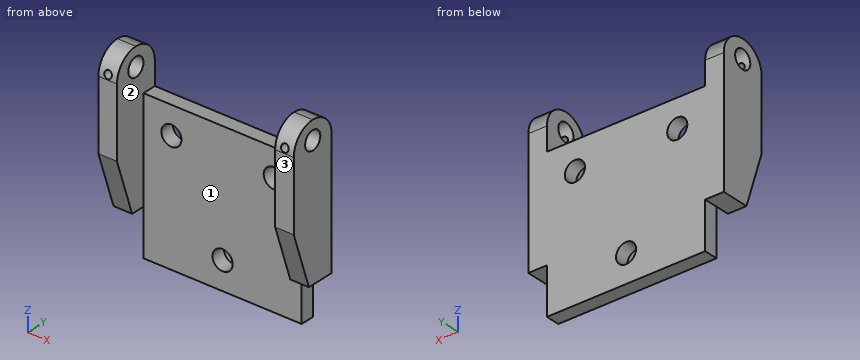
from build123d import *

# Parameters (mm, degrees)
F0_W         = 53.975
F0_H         = 50.8
F0_R         = 3.429
F1_DEPTH     = 4.7625
F2_W         = 6.35
F2_H         = 50.8
F3_DEPTH     = 15.875
F4_R         = 3.175
F5_DEPTH     = 6.35
F6_R         = 3.175
F7_DEPTH     = 6.35
F9_D         = 2.5781
F9_DEPTH     = 7.9375
F9_TIP       = 0.774539381
F10_T1_DEPTH = 46.0375
F10_T3_DEPTH = 46.0375
F11_SIZE2    = 19.05
F11_SIZE     = 6.35
F12_SIZE2    = 19.05
F12_SIZE     = 6.35


# Not quite as in the source:
# - a fillet or chamfer that OpenCascade refuses, or shapes differently, is made with other operations: its cross-section is extruded or revolved along the edge and cut away or added


with BuildPart() as f1:
    # F0 (on Front) → F1 (new body)
    with BuildSketch(Plane.XZ):
        with Locations((26.9875, 25.4)):
            Rectangle(F0_W, F0_H)
        with Locations((26.9875, 9.525)):
            Circle(F0_R, mode=Mode.SUBTRACT)
        with Locations((9.525, 41.275)):
            Circle(F0_R, mode=Mode.SUBTRACT)
        with Locations((44.45, 41.275)):
            Circle(F0_R, mode=Mode.SUBTRACT)
    extrude(amount=F1_DEPTH)

    # F2 (on Front) → F3 (join)
    with BuildSketch(Plane.XZ):
        with Locations((-3.175, 41.275)):
            Rectangle(F2_W, F2_H)
        with Locations((57.15, 41.275)):
            Rectangle(F2_W, F2_H)
    extrude(amount=F3_DEPTH)

    # F4 (on Right) → F5 (cut, through all)
    with BuildSketch(Plane.YZ):
        with Locations((-7.9375, 60.325)):
            Circle(F4_R)
    extrude(amount=-F5_DEPTH, mode=Mode.SUBTRACT)

    # F6 (on face) → F7 (cut)
    with BuildSketch(Plane.YZ.offset(60.325)):
        with Locations((-7.9375, 60.325)):
            Circle(F6_R)
    extrude(amount=-F7_DEPTH, mode=Mode.SUBTRACT)

    # F9
    with Locations(Plane.XZ.offset(15.875)):
        with Locations((-3.175, 60.325), (57.15, 60.325)):
            Hole(F9_D / 2, depth=F9_DEPTH)
            with Locations((0, 0, -(F9_DEPTH + F9_TIP / 2))):  # 118° drill point
                Cone(0, F9_D / 2, F9_TIP, mode=Mode.SUBTRACT)

    # F10: fillet of radius 7.9375 on 4 edges, made by hand

    # F10_s2 → F10_t1 (cut)
    with BuildSketch(Plane.YZ.offset(34.13125)):
        with BuildLine():
            ThreePointArc((-7.9375, 66.675), (-13.5501600757, 64.3501600757), (-15.875, 58.7375))
            Line((-15.875, 58.7375), (-15.875, 66.675))
            Line((-15.875, 66.675), (-7.9375, 66.675))
        make_face()
        with BuildLine():
            ThreePointArc((0, 58.7375), (-2.3248399243, 64.3501600757), (-7.9375, 66.675))
            Line((-7.9375, 66.675), (0, 66.675))
            Line((0, 66.675), (0, 58.7375))
        make_face()
    extrude(amount=F10_T1_DEPTH, mode=Mode.SUBTRACT)

    # F10_s4 → F10_t3 (cut)
    with BuildSketch(Plane.YZ.offset(-26.19375)):
        with BuildLine():
            ThreePointArc((-7.9375, 66.675), (-13.5501600757, 64.3501600757), (-15.875, 58.7375))
            Line((-15.875, 58.7375), (-15.875, 66.675))
            Line((-15.875, 66.675), (-7.9375, 66.675))
        make_face()
        with BuildLine():
            ThreePointArc((0, 58.7375), (-2.3248399243, 64.3501600757), (-7.9375, 66.675))
            Line((-7.9375, 66.675), (0, 66.675))
            Line((0, 66.675), (0, 58.7375))
        make_face()
    extrude(amount=F10_T3_DEPTH, mode=Mode.SUBTRACT)

    # F11
    f11_edges = [f1.edges().sort_by_distance(p)[0] for p in [
        (-3.175, -15.875, 15.875),
    ]]
    f11_side = f1.faces().sort_by_distance((-3.175, -7.9375, 15.875))[0]
    chamfer(f11_edges, length=F11_SIZE, length2=F11_SIZE2, reference=f11_side)

    # F12
    f12_edges = [f1.edges().sort_by_distance(p)[0] for p in [
        (57.15, -15.875, 15.875),
    ]]
    f12_side = f1.faces().sort_by_distance((57.15, -7.9375, 15.875))[0]
    chamfer(f12_edges, length=F12_SIZE, length2=F12_SIZE2, reference=f12_side)


solid = f1.part
The listing builds one solid part. Answer for the finished solid, in the listing's coordinates (mm). Face numbers are marked on the shaded views. A direction names the side the tool comes from. Round coordinates to 2 decimals unless told otherwise and drop trailing zeros. Order: outer loops, then holes, each group sorted by start corner. A loop starts at its lowest first (then second) coordinate and runs counter-clockwise, first axis right, second up. Notation, with made-up numbers: (82, 64) -> (94, 64) arc R17 cw to (94, 96) -> close; hole circle Ø5 at (62.5, -22.5). An arc over 180 degrees is marked (long way). One line per item, written item: value.
Item 1: Find section B-B, the plane y = -12. Give the vertices of the cut face in (x, z) (3 decimals), then the cut area to 3 significant figures.
Taken from the geometry:
outline: (-6.35, 23.3) -> (0, 23.3) -> (0, 65.557) -> (-6.35, 65.557) -> close; (53.975, 23.3) -> (60.325, 23.3) -> (60.325, 65.557) -> (53.975, 65.557) -> close; hole circle Ø2.578 at (-3.175, 60.325); hole circle Ø2.578 at (57.15, 60.325)
area: 526 mm2
Item 2: Given P1, Ø10, axis at x = 12, z = 54.5, coming from the -Y side; P2, Ø4, axis at y = -2.5, z = 6.5, coming from the +X side (3 decimals); P3, Ø5.5, axis at x = 44.45, z = 41.275, coming from the -Y side; P4, Ø5, axis at x = 27, y = -2, coming from the +Z side, each flat-ended and moving along its own axis, determine where each tip first touches the part or whether it passes through.
Taken from the geometry:
P1: stops at y = -4.76
P2: stops at x = 53.975
P3: passes through
P4: stops at z = 50.8
Item 3: Find section A-A, the plane x = 44.45. Give the vertices of the cut face in (y, z).
Taken from the geometry:
outline: (-4.76, 0) -> (0, 0) -> (0, 37.85) -> (-4.76, 37.85) -> close; (-4.76, 44.7) -> (0, 44.7) -> (0, 50.8) -> (-4.76, 50.8) -> close
Item 4: Straight lines are drawn through the part: L1, parallel to X at y = -14, z = 59 (3 decimals); L2, parallel to X at y = -0.75, z = 40.5 (3 decimals); L3, parallel to Z at x = 44.45, y = -3.1. For each, find the intervals that lie inside material, in ascending order.
Taken from the geometry:
L1: x = -6.35 to 0, 53.975 to 60.325
L2: x = -6.35 to 6.185, 12.865 to 41.11, 47.79 to 60.325
L3: z = 0 to 37.85, 44.7 to 50.8
Item 5: For the marked faces 1, 2 and 3, determine the directions among +Z, -Z, +X, -X, +Y, -Y from which every point of the face is accessible in a straight line to the end or side of a thin tool.
Taken from the geometry:
face 1: +Z, -Z, -Y
face 2: +Z, -Y
face 3: +Z, -Z, +X, -X, -Y
Item 6: Find section D-D, the plane y = -6. Give the vertices of the cut face in (x, z) (3 decimals), then the cut area to 3 significant figures.
Taken from the geometry:
outline: (-6.35, 15.875) -> (0, 15.875) -> (0, 57.81) -> (-6.35, 57.81) -> close; (-6.35, 62.84) -> (0, 62.84) -> (0, 66.435) -> (-6.35, 66.435) -> close; (53.975, 15.875) -> (60.325, 15.875) -> (60.325, 57.81) -> (53.975, 57.81) -> close; (53.975, 62.84) -> (60.325, 62.84) -> (60.325, 66.435) -> (53.975, 66.435) -> close
area: 578 mm2
